Autodesk Inventor part; units mm, degrees
ref_plane "Work Plane2" through (4.3439, -6.7266, 5.9732) normal (0, 0, 1) x (1, 0, 0)
ref_plane "YZ Plane" through (0, 0, 0) normal (1, 0, 0) x (0, 1, 0)
ref_plane "XZ Plane" through (0, 0, 0) normal (0, 1, 0) x (-1, 0, 0)
ref_plane "Work Plane1" through (25.9939, 2.4534, 2.2732) normal (0, 0, -1) x (-1, 0, 0)
sketch "Sketch1" plane through (25.9939, 2.4534, 2.2732) normal (0, 0, -1) x (-1, 0, 0)
  line L0 (21.65, -9.18) -> (-21.65, -9.18)
  line L1 (21.65, 9.18) -> (21.65, -9.18)
  line L2 (-21.65, 9.18) -> (21.65, 9.18)
  line L3 (-21.65, -9.18) -> (-21.65, 9.18)
  line L4 (24.65, 12.18) -> (24.65, -12.18)
  line L5 (24.65, -12.18) -> (-23.17, -12.18)
  line L6 (-23.17, 12.18) -> (24.65, 12.18)
  line L7 (-23.17, 3.98) -> (-23.17, -3.6)
  line L8 (-23.17, 12.18) -> (-23.17, -12.18)
  point P0 (25.9939, -2.4534)
  dimension "d0" = 3
extrude "Extrusion1" add sketch "Sketch1" along normal blind 2 contours L0 L3 L2 L1 | L4 L5 L8 L7 L6
sketch "Sketch2" plane through (25.9939, 2.4534, 2.2732) normal (0, 0, 1) x (1, 0, 0)
  line L0 (-24.65, 12.18) -> (-24.65, -12.18)
  line L1 (-24.65, -12.18) -> (23.17, -12.18)
  line L2 (21.65, 9.18) -> (-21.65, 9.18)
  line L3 (-21.65, 9.18) -> (-21.65, -9.18)
  line L4 (-21.65, -9.18) -> (21.65, -9.18)
  line L5 (21.65, -10.18) -> (-22.65, -10.18)
  line L6 (-22.65, -10.18) -> (-22.65, 10.18)
  line L7 (-22.65, 10.18) -> (21.65, 10.18)
  line L8 (21.65, 10.18) -> (21.65, -10.18)
  line L9 (-24.65, 12.18) -> (23.17, 12.18)
  line L10 (23.17, 12.18) -> (23.17, -12.18)
  line L11 (23.17, -12.18) -> (-24.65, -12.18)
  line L12 (-24.65, -12.18) -> (-24.65, 12.18)
  point P0 (-25.9939, -2.4534)
  dimension "d3" = 1
extrude "Extrusion2" add sketch "Sketch2" along normal blind 8
sketch "Sketch4" plane through (25.9939, 2.4534, 10.2732) normal (0, 0, 1) x (1, 0, 0)
  line L0 (21.65, 10.18) -> (21.65, -10.18)
  line L1 (23.17, 3.98) -> (13.97, 3.98) construction
  line L2 (13.97, -3.6) -> (23.17, -3.6) construction
  line L3 (21.65, 3.98) -> (23.17, 3.98)
  line L4 (23.17, 3.98) -> (23.17, -3.6)
  line L5 (23.17, -3.6) -> (21.65, -3.6)
  line L6 (21.65, -3.6) -> (21.65, 3.98)
  point P0 (-25.9939, -2.4534)
ref_plane "Work Plane2" through (4.3439, -6.7266, 5.9732) normal (0, 0, 1) x (1, 0, 0)
extrude "Extrusion4" cut sketch "Sketch4" against normal up to surface (4.3 mm away)
sketch "Sketch5" plane through (47.6439, -1.1466, 10.2732) normal (0, 1, 0) x (1, 0, 0)
  line L0 (1.52, 4.3) -> (0, 4.3)
  line L1 (0, 0) -> (0, 4.3)
  line L2 (1.52, 0) -> (0, 0)
  line L3 (1.52, 4.3) -> (1.52, 0)
  point P0 (-47.6439, 10.2732)
extrude "Extrusion5" cut sketch "Sketch5" against normal blind 0.3
sketch "Sketch6" plane through (47.6439, 6.4334, 10.2732) normal (0, -1, 0) x (1, 0, 0)
  line L0 (0, -4.3) -> (1.52, -4.3)
  line L1 (1.52, 0) -> (1.52, -4.3)
  line L2 (0, 0) -> (1.52, 0)
  line L3 (0, -4.3) -> (0, 0)
  point P0 (-47.6439, -10.2732)
extrude "Extrusion6" cut sketch "Sketch6" against normal blind 0.3
sketch "Sketch7" plane through (47.6439, 6.7334, 10.2732) normal (0, -1, 0) x (1, 0, 0)
  line L0 (1.52, 0) -> (1.52, -4.3)
  line L1 (0, 0) -> (1.52, 0)
  line L2 (0, -4.3) -> (0, 0)
  line L3 (0, 0) -> (1.52, 0)
  line L4 (1.52, 0) -> (1.52, -2)
  line L5 (1.52, -2) -> (0, -2)
  line L6 (0, -2) -> (0, 0)
  point P0 (-47.6439, -10.2732)
  dimension "d14" = 2
  dimension "d15" = 0
extrude "Extrusion7" cut sketch "Sketch7" against normal blind 4
sketch "Sketch8" plane through (25.9939, 2.4534, 2.2732) normal (0, 0, 1) x (1, 0, 0)
  line L0 (-22.65, 10.18) -> (-20.15, 10.18)
  line L1 (-20.15, 10.18) -> (-20.15, 7.68)
  line L2 (-20.15, 7.68) -> (-22.65, 7.68)
  line L3 (-22.65, 7.68) -> (-22.65, 10.18)
  line L4 (21.65, 10.18) -> (19.15, 10.18)
  line L5 (19.15, 10.18) -> (19.15, 7.68)
  line L6 (19.15, 7.68) -> (21.65, 7.68)
  line L7 (21.65, 7.68) -> (21.65, 10.18)
  line L8 (-22.65, -10.18) -> (-20.15, -10.18)
  line L9 (-20.15, -10.18) -> (-20.15, -7.68)
  line L10 (-20.15, -7.68) -> (-22.65, -7.68)
  line L11 (-22.65, -7.68) -> (-22.65, -10.18)
  line L12 (21.65, -10.18) -> (19.15, -10.18)
  line L13 (19.15, -10.18) -> (19.15, -7.68)
  line L14 (19.15, -7.68) -> (21.65, -7.68)
  line L15 (21.65, -7.68) -> (21.65, -10.18)
  point P0 (-25.9939, -2.4534)
  dimension "d18" = 2.5
  dimension "d19" = 2.5
  dimension "d20" = 2.5
  dimension "d21" = 2.5
  dimension "d22" = 2.5
  dimension "d23" = 2.5
extrude "Extrusion8" add sketch "Sketch8" along normal blind 2
fillet "Fillet1" radius 2 4 edges at (49.1639, 14.6334, 5.2732) (49.1639, -9.7266, 5.2732) (1.3439, 14.6334, 5.2732) (1.3439, -9.7266, 5.2732)
properties part number "NanoCaseBottom" material "ABS Plastic"
Here's how the part is built. I have some questions about the finished solid (model axes, mm). A direction names the side the tool comes from. Give positions to 0.01 mm unless a question says otherwise; leave off trailing zeros. Order: outer loops, then holes, each group sorted by start corner. A loop starts at its lowest first (then second) coordinate and runs counter-clockwise, first axis right, second up. Notation, with made-up numbers: M 17,-29 L 23,-29 A28 cw 23,-1 Z; hole C -10,84 d2. An arc over 180 degrees is marked long. Answer as a JSON object with one key per item and string values. Group by question number.
1) We'd pull the mould along Y, two halves only. Please class faces 4 (the flat face through (1.344, 3, 5)), 5 (the flat face through (25, -9.727, 5)), 6 (the flat face through (45.144, -6, 3)): pulls with the +Y half, pulls with the -Y half, needs draft (parallel to the pull), parting line crosses it, or undercut.
2) On a 3-axis mill with a long thin cutter (end or side, diameter ignored), from which of +Z, -Z, +X, -X, +Y, -Y can I reach the whole of each face in a straight line? I mean faces 1 (the flat face through (48, -1.447, 8)), 2 (the flat face through (25, 14.633, 5)), 3 (the flat face through (46, 11, 4.273)). Say none if no direction works.
3) Suppose I cut it at A-A, the plane z = 3. Write out the boundary of the cut face in (x, y).
4) Suppose I cut it at C-C, the plane y = 11.25. Write out the boundary of the cut face in (x, z), plus the area to 3 significant figures.
5) I'm going to push flat-ended pins straight in: pin 1 Ø0.5 at (x, y) = (48.5, 9.5) entering from +Z; pin 2 Ø1.7 at (x, z) = (49, 9.5) entering from -Y; pin 3 Ø4 at (x, y) = (23, 10.5) entering from +Z. Where does each tip first touch, or does it pass through?
6) Suppose I cut it at B-B, the plane x = 41. Write out the boundary of the cut face in (y, z), plus the area to 3 significant figures.
7) Suppose I cut it at D-D, the plane z = 7.25. Write out the boundary of the cut face in (x, y).
8) Please list where these lines run through material, in increasing order: L1, parallel to Y at x = 25.5, z = 5.5; L2, parallel to X at y = -6.75, z = 6.5; L3, parallel to Z at x = 9.5, y = 8.25. Write a range as [from, to].
Results found:
{
 "1": {"face 4": "needs draft", "face 5": "pulls with the -Y half", "face 6": "undercut"},
 "2": {"face 1": "+Z, +X", "face 2": "+Z, -Z, +X, -X, +Y", "face 3": "+Z"},
 "3": {"outline": "M 1.34,-7.73 A2 ccw 3.34,-9.73 L 47.16,-9.73 A2 ccw 49.16,-7.73 L 49.16,12.63 A2 ccw 47.16,14.63 L 3.34,14.63 A2 ccw 1.34,12.63 Z; hole M 3.34,-5.23 L 5.84,-5.23 L 5.84,-7.73 L 45.14,-7.73 L 45.14,-5.23 L 47.64,-5.23 L 47.64,10.13 L 45.14,10.13 L 45.14,12.63 L 5.84,12.63 L 5.84,10.13 L 3.34,10.13 Z"},
 "4": {"outline": "M 1.34,0.27 L 49.16,0.27 L 49.16,10.27 L 47.64,10.27 L 47.64,4.27 L 45.14,4.27 L 45.14,2.27 L 5.84,2.27 L 5.84,4.27 L 3.34,4.27 L 3.34,10.27 L 1.34,10.27 Z", "area": "134 mm²"},
 "5": {"pin 1": "z = 8.27", "pin 2": "y = -9.47", "pin 3": "z = 2.27"},
 "6": {"outline": "M -9.73,0.27 L 14.63,0.27 L 14.63,10.27 L 12.63,10.27 L 12.63,2.27 L -7.73,2.27 L -7.73,10.27 L -9.73,10.27 Z", "area": "80.7 mm²"},
 "7": {"outline": "M 1.34,-7.73 A2 ccw 3.34,-9.73 L 47.16,-9.73 A2 ccw 49.16,-7.73 L 49.16,-1.45 L 47.64,-1.45 L 47.64,-7.73 L 3.34,-7.73 L 3.34,12.63 L 47.64,12.63 L 47.64,6.73 L 49.16,6.73 L 49.16,12.63 A2 ccw 47.16,14.63 L 3.34,14.63 A2 ccw 1.34,12.63 Z"},
 "8": {"L1": "[-9.73, -7.73], [12.63, 14.63]", "L2": "[1.34, 3.34], [47.64, 49.16]", "L3": "[0.27, 2.27]"}
}
